```python
from build123d import *

# Parameters (mm, degrees)
F1_DEPTH = 114.3
F3_DEPTH = 114.3
F5_DEPTH = 114.301


with BuildPart() as f1:
    # F0 (on Front) → F1 (new body)
    with BuildSketch(Plane.XZ):
        Polygon((38.1, 0), (0, 0), (0, -12.7), (152.4, -12.7), (152.4, 0), (114.3, 0), (114.3, 98.425), (38.1, 98.425), align=None)
    extrude(amount=F1_DEPTH)

    # F2 (on face) → F3 (cut)
    with BuildSketch(Plane.XZ.offset(114.3)):
        with BuildLine():
            Line((107.95, 98.425), (44.45, 98.425))
            ThreePointArc((44.45, 98.425), (76.2, 89.917613), (107.95, 98.425))
        make_face()
    extrude(amount=-F3_DEPTH, mode=Mode.SUBTRACT)

    # F4 (on face) → F5 (cut, through all)
    with BuildSketch(Plane.XZ.offset(114.3)):
        with BuildLine():
            ThreePointArc((107.95, 98.425), (76.2, 89.917613), (44.45, 98.425))
            ThreePointArc((44.45, 98.425), (76.2, 66.496828), (107.95, 98.425))
        make_face()
    extrude(amount=-F5_DEPTH, mode=Mode.SUBTRACT)


solid = f1.part
```
Part model, mm, in its own coordinate system. A direction names the side the tool comes from. Round coordinates to 2 decimals unless told otherwise and drop trailing zeros. Write each loop counter-clockwise with the first axis right and the second up, starting at its lowest first coordinate (ties: lowest second). Pieces come first, ordered by that corner, then holes. Notation, with made-up numbers: (38, -9.5) -> (47, -9.5) arc R25 cw to (47, 5.5) -> close; hole circle Ø5 at (-19.75, 14.5). An arc over 180 degrees is marked (long way). Return JSON: item names as keys, results as strings. Group by question number.
Q1. Saw through at C-C on z = 22. Write the cut outline in (x, y), plus the area to 3 significant figures.
Q2. Mould opens along X. For faces 4 (the flat face through (152.4, -56, -6)), 5 (the flat face through (75, 0, 31)), 6 (the cylindrical face through (75.499, -57.95, 66.505)) say: pulls with the +X half, pulls with the -X half, needs draft (parallel to the pull), parting line crosses it, or undercut.
Q3. Probe L1, parallel to X at y = -49, z = 61.5; L2, parallel to Z at x = 13, y = -58.5; L3, parallel to X at y = -96, z = 90.5. List the from-to ranges inside material, lowest first. Write a range as [from, to].
Q4. Pin check, flat tips, straight feed: pin 1 (6 mm diameter, centred on y = -84, z = 35, fed in from +X); pin 2 (2 mm diameter, centred on y = -72.5, z = 15.5, fed in from -X); pin 3 (19 mm diameter, centred on x = 126, y = -62, fed in from +Z). Stop position of each tip, or through.
Q5. Saw through at B-B on x = 76.2. Write the cut outline in (y, z).
Q6. Which spindle directions (+Z, -Z, +X, -X, +Y, -Y) get a long thin tool onto all of the face, cutting with end or side? Do faces 1 (the flat face through (111, -56, 98.425)), 2 (the flat face through (134, -56, 0)), 3 (the flat face through (19, -56, 0)). Say none if no direction does.
Answer:
{
 "1": {"outline": "(38.1, -114.3) -> (114.3, -114.3) -> (114.3, 0) -> (38.1, 0) -> close", "area": "8,710 mm2"},
 "2": {"face 4": "pulls with the +X half", "face 5": "needs draft", "face 6": "undercut"},
 "3": {"L1": "[38.1, 114.3]", "L2": "[-12.7, 0]", "L3": "[38.1, 45.41], [106.99, 114.3]"},
 "4": {"pin 1": "x = 114.3", "pin 2": "x = 38.1", "pin 3": "z = 0"},
 "5": {"outline": "(-114.3, -12.7) -> (0, -12.7) -> (0, 66.5) -> (-114.3, 66.5) -> close"},
 "6": {"face 1": "+Z, +X, -X, +Y, -Y", "face 2": "+Z, +X, +Y, -Y", "face 3": "+Z, -X, +Y, -Y"}
}
